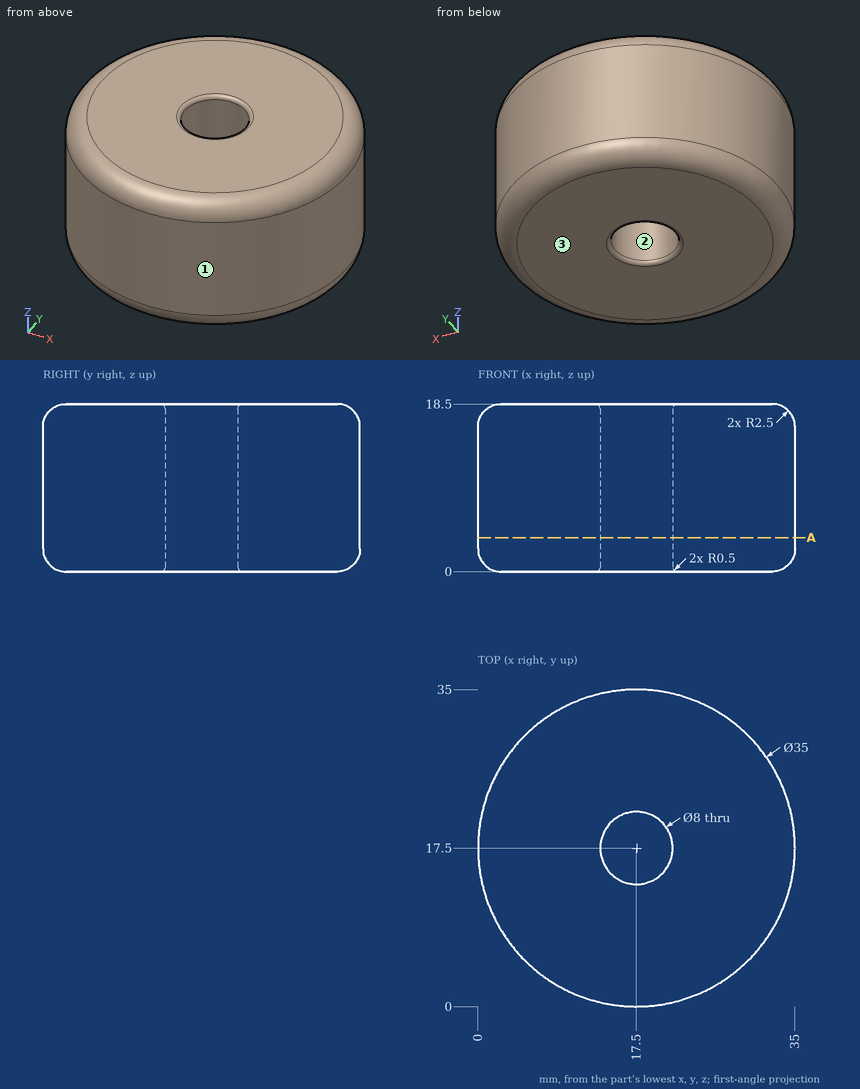
Job drawing, mm, ordinate dimensions from the low corner. One solid piece. Round coordinates to 2 decimals unless told otherwise and drop trailing zeros. Loops run counter-clockwise (first coordinate to the right, second up) from the corner with the lowest first, then second, coordinate; pieces in that order, holes last.
(1) Wall check: line 1 along Y through (x, z) = (17.5, 12); line 2 along X through (y, z) = (14.5, 11.5); line 3 along Y through (x, z) = (20, 9). Give the ranges that are in metal, low to high.
(2) Cut at A-A (z = 3.75). Give the cut face in (x, y), plus the area to 3 significant figures.
(3) Two-plate mould, pull along X, no slides. Class the marked faces 1, 2 and 3: +X half, -X half, draft (parallel to the pull), parting line (faces both ways), or undercut.
(4) Drop flat-ended pins along their axis: pin 1 (8 mm diameter, centred on x = 26.5, y = 15.5, fed in from -Z); pin 2 (1 mm diameter, centred on y = 27, z = 5.5, fed in from +X); pin 3 (3 mm diameter, centred on x = 28, z = 11.5, fed in from -Y); pin 4 (2 mm diameter, centred on y = 6, z = 4.5, fed in from -X). Give the stop position or say it passes through.
Findings below:
1. line 1: y = 0 to 13.5, 21.5 to 35
1. line 2: x = 0.26 to 14.85, 20.15 to 34.74
1. line 3: y = 0.18 to 14.38, 20.62 to 34.82
2. outline: circle Ø35 at (17.5, 17.5); hole circle Ø8 at (17.5, 17.5)
2. area: 912 mm2
3. face 1: parting line
3. face 2: undercut
3. face 3: draft
4. pin 1: stops at z = 0
4. pin 2: stops at x = 32.51
4. pin 3: stops at y = 2.49
4. pin 4: stops at x = 3.5
